Design review of the part built by this model. Coordinates are the model's own, in mm. A direction names the side the tool comes from. Give positions to 0.01 mm unless a question says otherwise; leave off trailing zeros. Write each loop counter-clockwise with the first axis right and the second up, starting at its lowest first coordinate (ties: lowest second). Pieces come first, ordered by that corner, then holes. Notation, with made-up numbers: (47.25, -32.5) -> (74.25, -32.5) arc R24 ccw to (74.25, -19.5) -> close; hole circle Ø5 at (56.25, 30.5). An arc over 180 degrees is marked (long way). Write each question's results on one line, items separated by ' | '. Start each with the question number.
(1) For faces 1 (the face through (-5.158, -3.955, 4.451)), 2 (the face through (3, 3, 8)), 3 (the face through (0, 0, 2)), list the 3-axis set-ups (+Z, -Z, +X, -X, +Y, -Y) from which the entire face can be reached by the end or side of a thin tool; tool diameter is ignored.
(2) To check wall thickness, follow probe 1 along Z at (x, y) = (-1.5, -2.5); probe 2 along Z at (x, y) = (-4.25, 0.5); probe 3 along Y at (x, z) = (0, 24.5). State the ranges of each line that lie inside material, in increasing order.
(3) Take a section at C-C (z = 7.25). State the section outline as (x, y) points.
(4) Clearance check with flat-ended pins moving along their axes: pin 1 (3 mm diameter, centred on y = 0, z = 20.5, fed in from +X); pin 2 (3 mm diameter, centred on x = 1, y = -1, fed in from -Z); pin 3 (4 mm diameter, centred on y = -4, z = 14.5, fed in from +X). State where each tip first meets the part, or that it passes through.
(5) Mouldability with a two-part tool opening along Y and no side actions: class faces 4 (the face through (-0.86, -3.874, 17.446)), 5 (the face through (0, 0, 28)), 6 (the face through (0, -3.031, 1)) as released by +Y, released by -Y, zero draft, split by the parting line, or undercut.
(6) Take a section at A-A (x = 0). State the section outline as (y, z) points, plus the area to 3 significant figures.
(7) Take a section at B-B (z = 16.5). State the section outline as (x, y) points, plus the area to 3 significant figures.
from build123d import *

# Parameters (mm, degrees)
SKETCH_1_R               = 6.5
EXTRUDE_1_DEPTH          = 8
SKETCH_2_R               = 4
EXTRUDE_2_DEPTH          = 20
FILLET_1_R               = 1
CUT_EXTRUDE_1_DEPTH      = 30.470324079
CUT_EXTRUDE_1_DEPTH_BACK = 2


# Read off the part's stored shape, not the designer's step: 5/16-18 机械螺纹 螺柱1
with BuildPart() as part:
    # 草图1 → 凸台-拉伸1 (new body)
    with BuildSketch(Plane.XY):
        Circle(SKETCH_1_R)
    extrude(amount=EXTRUDE_1_DEPTH)

    # 草图2 → 凸台-拉伸2 (add)
    with BuildSketch(Plane.XY.offset(8)):
        Circle(SKETCH_2_R)
    extrude(amount=EXTRUDE_2_DEPTH)

    # 5/16-18 机械螺纹 螺柱1 outline → 5/16-18 机械螺纹 螺柱1 (revolve, cut)
    with BuildSketch(Plane.XZ):
        Polygon((4, 28), (3.12928, 28), (3.96875, 27.16053), (3.96875, 8), (4, 8), align=None)
    revolve(axis=Axis((0, 0, 0), (0, 0, 1)), mode=Mode.SUBTRACT)

    # 圆角1
    fillet_1_edges = [part.edges().sort_by_distance(p)[0] for p in [
        (-6.5, 0, 0),
    ]]
    fillet(fillet_1_edges, radius=FILLET_1_R)

    # 草图4 → 切除-拉伸1 (cut, two sides: drawn at the far end of the back side and taken through both)
    with BuildSketch(Plane(origin=(0, 0, 0), x_dir=(-1, 0, 0), z_dir=(0, 0, -1)).offset(-CUT_EXTRUDE_1_DEPTH_BACK)):
        Polygon((3.5, 0), (1.75, 3.031088913), (-1.75, 3.031088913), (-3.5, 0), (-1.75, -3.031088913), (1.75, -3.031088913), align=None)
    extrude(amount=CUT_EXTRUDE_1_DEPTH + CUT_EXTRUDE_1_DEPTH_BACK, mode=Mode.SUBTRACT)


solid = part.part
Report:
1) face 1: +Z, -Z | face 2: +Z | face 3: -Z
2) probe 1: 2 to 28 | probe 2: 0 to 8 | probe 3: -3.97 to 3.97
3) outline: circle Ø13 at (0, 0)
4) pin 1: x = 3.97 | pin 2: z = 2 | pin 3: x = 3.43
5) face 4: split by the parting line | face 5: zero draft | face 6: undercut
6) outline: (-6.5, 1) arc R1 ccw to (-5.5, 0) -> (-3.03, 0) -> (-3.03, 2) -> (3.03, 2) -> (3.03, 0) -> (5.5, 0) arc R1 ccw to (6.5, 1) -> (6.5, 8) -> (3.97, 8) -> (3.97, 27.16) -> (3.13, 28) -> (-3.13, 28) -> (-3.97, 27.16) -> (-3.97, 8) -> (-6.5, 8) -> close | area: 249 mm2
7) outline: circle Ø7.94 at (0, 0) | area: 49.5 mm2
